Check sheet for the modelled part. Datum: model origin and axes. Units: mm. A direction names the side the tool comes from. Give positions to 0.01 mm unless a question says otherwise; leave off trailing zeros. Loops run counter-clockwise (first coordinate to the right, second up) from the corner with the lowest first, then second, coordinate; pieces in that order, holes last. Notation, with made-up numbers: (61.25, 74) -> (101.25, 74) arc R17 ccw to (101.25, 87) -> close; hole circle Ø2 at (35, 3). An arc over 180 degrees is marked (long way). Write each question's results on one line, items separated by ' | '. Start each with the question number.
1. Material ranges on L1, parallel to Y at x = -2608.5, z = 352; L2, parallel to X at y = 400.5, z = 369; L3, parallel to Y at x = -1250, z = 302.5, recorded low to high. Write a range as from..to.
2. Cross-section at A-A on x = -2374.5. Record the boundary of the cut face in (y, z).
3. Cross-section at B-B on z = 182. Record the boundary of the cut face in (x, y), and give its area (3 significant figures).
4. Cross-section at D-D on z = 568.5. Record the boundary of the cut face in (x, y).
5. Gauge pin test, flat ends, axial feed: pin 1 Ø10 at (x, z) = (-1157, 295) entering from +Y; pin 2 Ø8 at (y, z) = (176.5, 470) entering from -X; pin 3 Ø6 at (y, z) = (605.5, 132) entering from +X. Record the tip position at first contact, or that the pin passes through.
6. Cross-section at C-C on y = 474.5. Record the boundary of the cut face in (x, z).
7. Mould release check, pull along Y, two halves, no side actions. Record for faces 1 (the face through (-2518.376, 929, 152)), 2 (the face through (-2394, 779.006, 368)), 3 (the face through (-2231, 1083.806, 301)): +Y half, -Y half, draft (parallel to the pull), parting line (faces both ways), or undercut.
8. Tool access check on faces 4 (the face through (-2111.976, 453, 301)), 5 (the face through (-534, 453, 152.4)), 6 (the face through (-834, 779.006, 301)), 7 (the face through (-850, 118.606, 301)), 8 (the face through (-2669, 934, 307.34)). Record the directions out of +Z, -Z, +X, -X, +Y, -Y that give a thin tool (end or side, any length) a straight path to the whole face; none if there is none.
from build123d import *

# Parameters (mm, degrees)
Y_KSEKLIK_EKSTR_ZYON3_DEPTH = 609.6
IZIM2_W                     = 508
IZIM2_H                     = 660.4
KES_EKSTR_ZYON1_DEPTH       = 152.4
IZIM3_W                     = 304.8
IZIM3_H                     = 304.8
KES_EKSTR_ZYON2_DEPTH       = 307.34


with BuildPart() as part:
    # Çizim1 → Yükseklik-Ekstrüzyon3 (new body)
    with BuildSketch(Plane.XY):
        Polygon((-283.176149051, 779.0060667), (-1400.776149051, 779.0060667), (-1654.776149051, 1083.8060667), (-2823.176149051, 1083.8060667), (-2823.176149051, 779.0060667), (-2111.976149051, 779.0060667), (-2111.976149051, 118.6060667), (-2823.176149051, 118.6060667), (-2823.176149051, -186.1939333), (-1654.776149051, -186.1939333), (-1400.776149051, 118.6060667), (-283.176149051, 118.6060667), align=None)
    extrude(amount=Y_KSEKLIK_EKSTR_ZYON3_DEPTH)

    # Çizim2 → Kes-Ekstrüzyon1 (cut)
    with BuildSketch(Plane(origin=(0, 0, 0), x_dir=(-1, 0, 0), z_dir=(0, 0, -1))):
        with Locations((537.176149051, 448.8060667)):
            Rectangle(IZIM2_W, IZIM2_H)
    extrude(amount=-KES_EKSTR_ZYON1_DEPTH, mode=Mode.SUBTRACT)

    # Çizim3 → Kes-Ekstrüzyon2 (cut)
    with BuildSketch(Plane(origin=(0, 0, 0), x_dir=(-1, 0, 0), z_dir=(0, 0, -1))):
        with Locations((2670.776149051, -33.7939333)):
            Rectangle(IZIM3_W, IZIM3_H)
        with Locations((2670.776149051, 931.4060667)):
            Rectangle(IZIM3_W, IZIM3_H)
    extrude(amount=-KES_EKSTR_ZYON2_DEPTH, mode=Mode.SUBTRACT)


solid = part.part
Geometry says:
1) L1: -186.19..118.61, 779.01..1083.81 | L2: -2111.98..-283.18 | L3: 118.61..779.01
2) outline: (-186.19, 0) -> (118.61, 0) -> (118.61, 609.6) -> (-186.19, 609.6) -> close; (779.01, 0) -> (1083.81, 0) -> (1083.81, 609.6) -> (779.01, 609.6) -> close
3) outline: (-2518.38, -186.19) -> (-1654.78, -186.19) -> (-1400.78, 118.61) -> (-283.18, 118.61) -> (-283.18, 779.01) -> (-1400.78, 779.01) -> (-1654.78, 1083.81) -> (-2518.38, 1083.81) -> (-2518.38, 779.01) -> (-2111.98, 779.01) -> (-2111.98, 118.61) -> (-2518.38, 118.61) -> close | area: 1,810,000 mm^2
4) outline: (-2823.18, -186.19) -> (-1654.78, -186.19) -> (-1400.78, 118.61) -> (-283.18, 118.61) -> (-283.18, 779.01) -> (-1400.78, 779.01) -> (-1654.78, 1083.81) -> (-2823.18, 1083.81) -> (-2823.18, 779.01) -> (-2111.98, 779.01) -> (-2111.98, 118.61) -> (-2823.18, 118.61) -> close
5) pin 1: y = 779.01 | pin 2: x = -2111.98 | pin 3: x = -791.18
6) outline: (-2111.98, 0) -> (-791.18, 0) -> (-791.18, 152.4) -> (-283.18, 152.4) -> (-283.18, 609.6) -> (-2111.98, 609.6) -> close
7) face 1: draft | face 2: undercut | face 3: +Y half
8) face 4: +Z, -Z, -X | face 5: -Z, +X, +Y, -Y | face 6: +Z, -Z, +X, +Y | face 7: +Z, -Z, +X, -Y | face 8: -Z, -X, +Y, -Y
